Could you check a few things on this drawing? It's one solid part, dimensions in mm from its lowest x, y, z. A direction names the side the tool comes from. Give positions to 0.01 mm unless a question says otherwise; leave off trailing zeros. Order: outer loops, then holes, each group sorted by start corner. A loop starts at its lowest first (then second) coordinate and runs counter-clockwise, first axis right, second up. Notation, with made-up numbers: (-8, -20.75) - (40, -20.75) arc R22 cw to (40, -4.75) - close; hole circle Ø11 at (74.5, 13). An arc over 180 degrees is marked (long way). Answer as CSV lines item,"result".
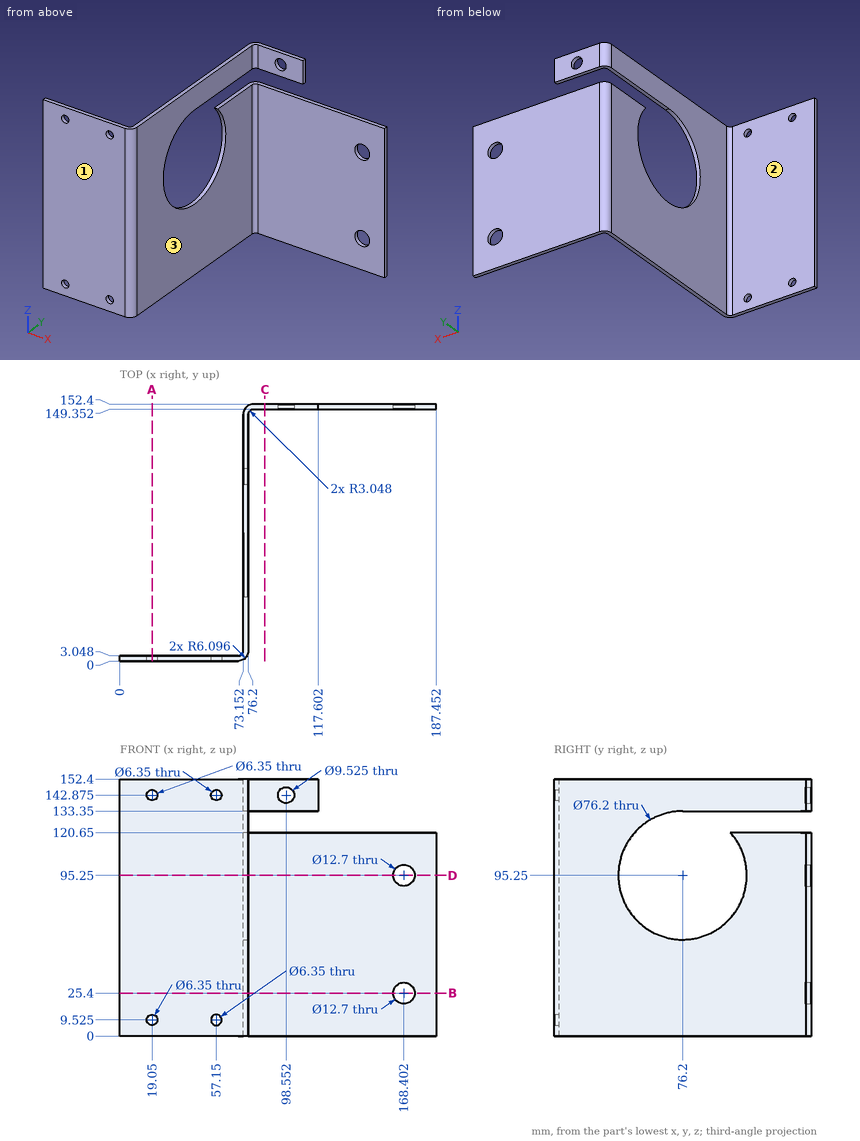
1) Which directions (+Z, -Z, +X, -X, +Y, -Y) give clear straight access to the entire face, cutting with the end or side of a thin tool? Please do the marked faces 1, 2 and 3.
Answer block:
face 1,"+Z, -Z, +X, -X, -Y"
face 2,"+Z, -Z, -X, +Y"
face 3,"+Z, -Z, +X, -Y"
2) I want a section at B-B on z = 25.4. Write out the boundary of the cut face in (x, y), plus the area to 3 significant figures.
Answer block:
outline,"(0, 0) - (70.1, 0) arc R6.1 ccw to (76.2, 6.1) - (76.2, 146.3) arc R3.05 cw to (79.25, 149.35) - (162.05, 149.35) - (162.05, 152.4) - (79.25, 152.4) arc R6.1 ccw to (73.15, 146.3) - (73.15, 6.1) arc R3.05 cw to (70.1, 3.05) - (0, 3.05) - close; (174.75, 149.35) - (187.45, 149.35) - (187.45, 152.4) - (174.75, 152.4) - close"
area,"976 mm2"
3) I want a section at A-A on x = 19.05. Write out the boundary of the cut face in (y, z), plus the area to 3 significant figures.
Answer block:
outline,"(0, 0) - (3.05, 0) - (3.05, 6.35) - (0, 6.35) - close; (0, 12.7) - (3.05, 12.7) - (3.05, 139.7) - (0, 139.7) - close; (0, 146.05) - (3.05, 146.05) - (3.05, 152.4) - (0, 152.4) - close"
area,"426 mm2"
4) I'm going to push flat-ended pins straight in: P1, Ø2, axis at x = 114.5, z = 87, coming from the -Y side; P2, Ø24, axis at x = 146.5, y = 132.5, coming from the +Z side; P3, Ø3, axis at y = 122, z = 118, coming from the -X side; P4, Ø10, axis at x = 79.5, z = 120, coming from the -Y side. Where does each tip first touch, or does it pass through?
Answer block:
P1,"y = 149.35"
P2,"through"
P3,"x = 73.15"
P4,"y = 1.87"
5) I need wall thicknesses on line 1 along Z through (x, y) = (19, 1); line 2 along Y through (x, z) = (31, 8.5); line 3 along Y through (x, z) = (139, 27.5). Which ranges of each line are inside material? Lowest first, please. Write a range as [from, to].
Answer block:
line 1,"[0, 6.35], [12.7, 139.7], [146.05, 152.4]"
line 2,"[0, 3.05]"
line 3,"[149.35, 152.4]"
6) I want a section at C-C on x = 86. Write out the boundary of the cut face in (y, z), plus the area to 3 significant figures.
Answer block:
outline,"(149.35, 0) - (152.4, 0) - (152.4, 120.65) - (149.35, 120.65) - close; (149.35, 133.35) - (152.4, 133.35) - (152.4, 152.4) - (149.35, 152.4) - close"
area,"426 mm2"
7) I want a section at D-D on z = 95.25. Write out the boundary of the cut face in (x, y).
Answer block:
outline,"(0, 0) - (70.1, 0) arc R6.1 ccw to (76.2, 6.1) - (76.2, 38.1) - (73.15, 38.1) - (73.15, 6.1) arc R3.05 cw to (70.1, 3.05) - (0, 3.05) - close; (73.15, 114.3) - (76.2, 114.3) - (76.2, 146.3) arc R3.05 cw to (79.25, 149.35) - (162.05, 149.35) - (162.05, 152.4) - (79.25, 152.4) arc R6.1 ccw to (73.15, 146.3) - close; (174.75, 149.35) - (187.45, 149.35) - (187.45, 152.4) - (174.75, 152.4) - close"
